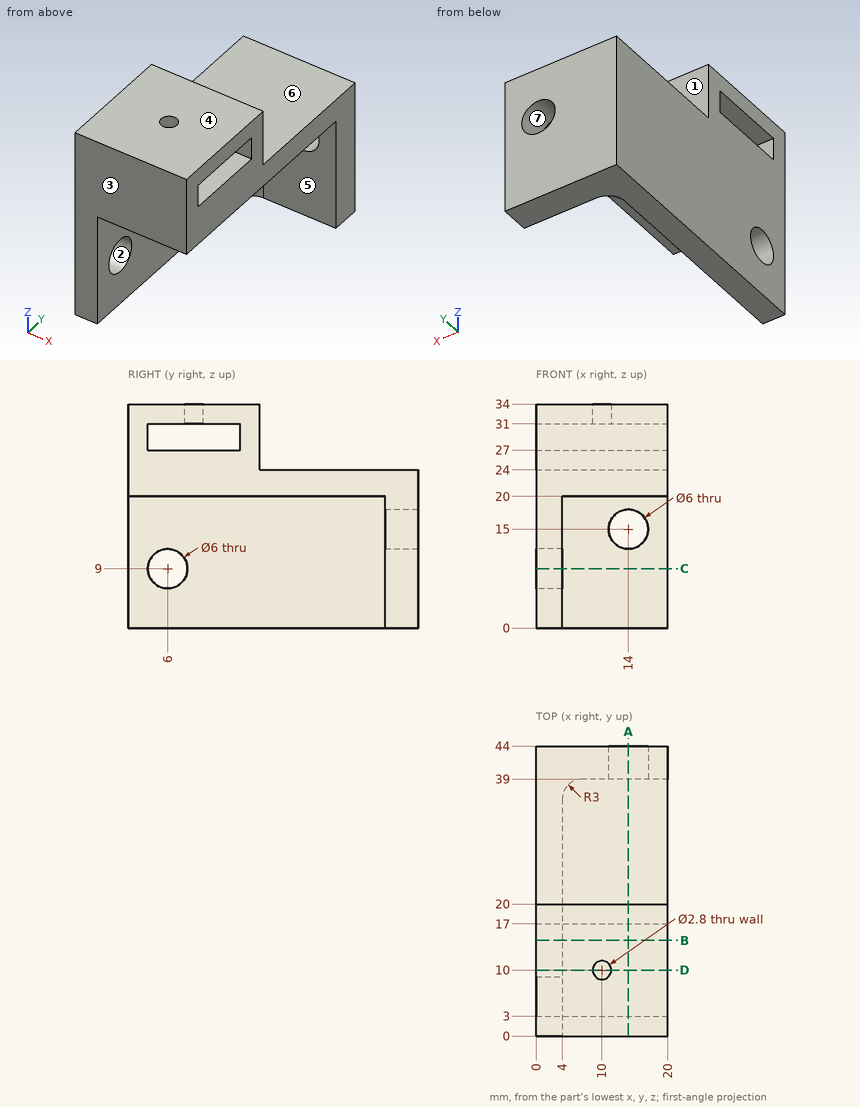
Study the drawing (mm; zero at the part's minimum x, y, z) and answer. A direction names the side the tool comes from. Round coordinates to 2 decimals unless told otherwise and drop trailing zeros. Write each loop counter-clockwise with the first axis right and the second up, starting at its lowest first coordinate (ties: lowest second). Pieces come first, ordered by that corner, then holes. Notation, with made-up numbers: (68, 25) -> (117, 25) arc R22 ccw to (117, 41) -> close; hole circle Ø7 at (83, 11). An arc over 180 degrees is marked (long way). Use CSV: the item, a comma, the result in double quotes. Start each with the question number.
(1) Section C-C on z = 9 is taken. Give the vertices of the cut face in (x, y).
(2) Each of these flat-tipped pins is pushed along its axis until it touches: pin 1 (4 mm diameter, centred on y = 19, z = 11.5, fed in from +X); pin 2 (6 mm diameter, centred on y = 33, z = 27.5, fed in from -X); pin 3 (10.5 mm diameter, centred on x = 11, z = 6.5, fed in from -Y); pin 4 (2 mm diameter, centred on x = 13.5, y = 25.5, fed in from -Z). Where does it stop, or does it pass through?
(3) Section D-D on y = 10 is taken. Give the vertices of the cut face in (x, z).
(4) The mould has two halves that part along Y. Classify the marked faces 1, 2, 3 and 4: released by +Y, released by -Y, zero draft, split by the parting line, or undercut.
(5) Section A-A on x = 14 is taken. Give the vertices of the cut face in (y, z), then the cut area to 3 significant figures.
(6) Which of the six approach directions +Z, -Z, +X, -X, +Y, -Y give full straight-line access (tool end or side, diameter ignored) to the marked faces 5, 6 and 7?
(7) Consider L1, parallel to Y at x = 1.8, z = 9; L2, parallel to Y at x = 10, z = 33.3; L3, parallel to Z at x = 10.5, y = 8. Determine where each line is inside the solid, lowest interval first. Write a range as from..to.
(8) Section B-B on y = 14.5 is taken. Give the vertices of the cut face in (x, z), then the cut area to 3 significant figures.
A:
1,outline,"(0, 0) -> (4, 0) -> (4, 3) -> (0, 3) -> close; (0, 9) -> (4, 9) -> (4, 36) arc R3 cw to (7, 39) -> (20, 39) -> (20, 44) -> (0, 44) -> close"
2,pin 1,"stops at x = 4"
2,pin 2,"passes through"
2,pin 3,"stops at y = 38.73"
2,pin 4,"stops at z = 20"
3,outline,"(0, 0) -> (4, 0) -> (4, 20) -> (20, 20) -> (20, 27) -> (0, 27) -> close; (0, 31) -> (8.6, 31) -> (8.6, 34) -> (0, 34) -> close; (11.4, 31) -> (20, 31) -> (20, 34) -> (11.4, 34) -> close"
4,face 1,"released by +Y"
4,face 2,"undercut"
4,face 3,"released by -Y"
4,face 4,"zero draft"
5,outline,"(0, 20) -> (39, 20) -> (39, 18) -> (44, 18) -> (44, 24) -> (20, 24) -> (20, 34) -> (0, 34) -> close; (39, 0) -> (44, 0) -> (44, 12) -> (39, 12) -> close; hole (3, 27) -> (17, 27) -> (17, 31) -> (3, 31) -> close"
5,area,"390 mm²"
6,face 5,"-Z, +X, -Y"
6,face 6,"+Z, +X, -X, +Y"
6,face 7,"+Y, -Y"
7,L1,"y = 0..3, 9..44"
7,L2,"y = 0..8.6, 11.4..20"
7,L3,"z = 20..27, 31..34"
8,outline,"(0, 0) -> (4, 0) -> (4, 20) -> (20, 20) -> (20, 27) -> (0, 27) -> close; (0, 31) -> (20, 31) -> (20, 34) -> (0, 34) -> close"
8,area,"280 mm²"
